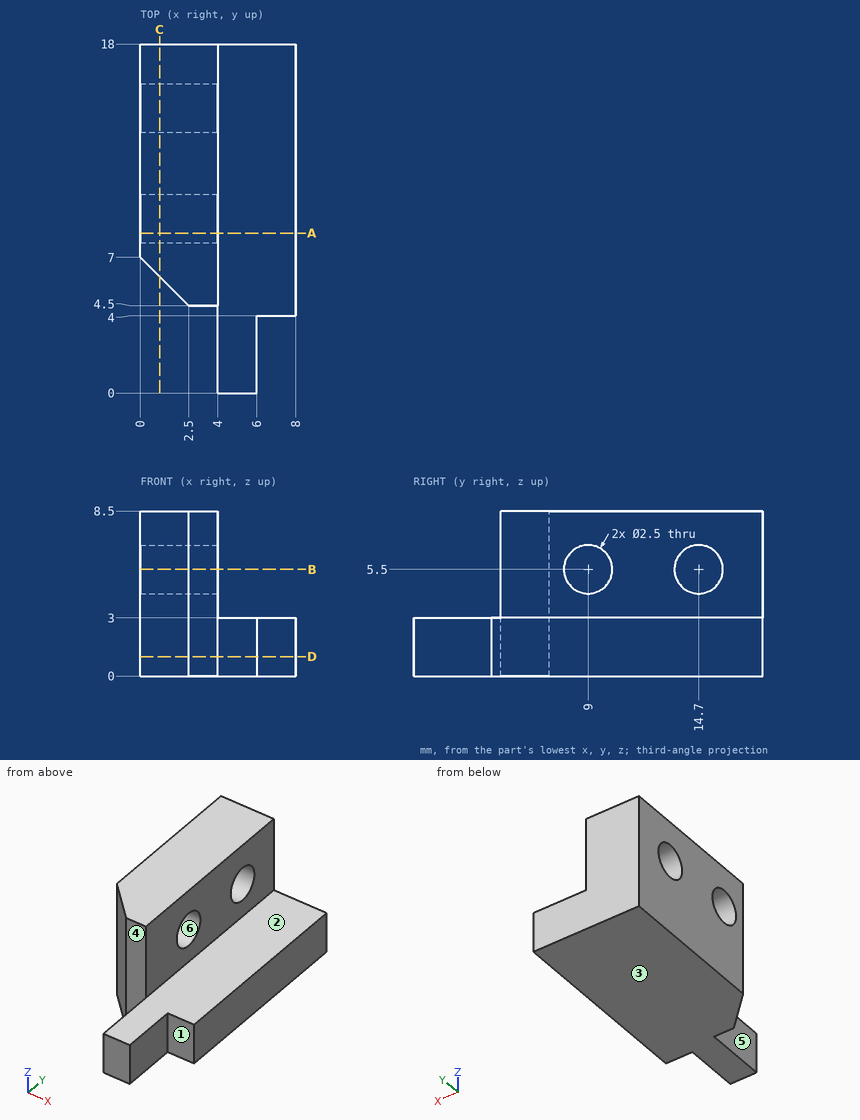
Part print with two shaded views. Sizes in mm from the minimum x, y, z corner. A direction names the side the tool comes from. Round coordinates to 2 decimals unless told otherwise and drop trailing zeros. Loops run counter-clockwise (first coordinate to the right, second up) from the corner with the lowest first, then second, coordinate; pieces in that order, holes last.
Item 1: Drill centre lines: line 1 along Y through (x, z) = (2.7, 5.5); line 2 along Y through (x, z) = (1, 5.5); line 3 along Y through (x, z) = (1, 2). Where is each one in solid material? Low to high.
Item 2: Which spindle directions (+Z, -Z, +X, -X, +Y, -Y) get a long thin tool onto all of the face, cutting with end or side? Do the marked faces 1, 2 and 3. Say none if no direction does.
Item 3: Saw through at A-A (y = 8.25). List the corners of the cut face in (x, z).
Item 4: Pin check, flat tips, straight feed: P1, Ø2.5, axis at y = 2.5, z = 1.5, coming from the +X side; P2, Ø0.8, axis at x = 3, z = 4.5, coming from the -Y side; P3, Ø2, axis at y = 9, z = 5.5, coming from the -X side; P4, Ø4.5, axis at y = 13.5, z = 7, coming from the +X side. Stop position of each tip, or through.
Item 5: Saw through at C-C (x = 1). List the corners of the cut face in (y, z).
Item 6: Two-plate mould, pull along Y, no slides. Class the marked faces 4, 5 and 6: released by +Y, released by -Y, zero draft, split by the parting line, or undercut.
Item 7: Saw through at B-B (z = 5.5). List the corners of the cut face in (x, y).
Item 8: Saw through at D-D (z = 1). List the corners of the cut face in (x, y), then the cut area to 3 significant figures.
Worked answers:
1. line 1: y = 4.5 to 7.75, 10.25 to 13.45, 15.95 to 18
1. line 2: y = 6 to 7.75, 10.25 to 13.45, 15.95 to 18
1. line 3: y = 6 to 18
2. face 1: +Z, -Z, +X, -Y
2. face 2: +Z, +X, +Y, -Y
2. face 3: -Z, +X, -X, +Y, -Y
3. outline: (0, 0) - (8, 0) - (8, 3) - (4, 3) - (4, 4.5) - (0, 4.5) - close; (0, 6.5) - (4, 6.5) - (4, 8.5) - (0, 8.5) - close
4. P1: stops at x = 6
4. P2: stops at y = 4.5
4. P3: passes through
4. P4: stops at x = 4
5. outline: (6, 0) - (18, 0) - (18, 8.5) - (6, 8.5) - close; hole circle Ø2.5 at (9, 5.5); hole circle Ø2.5 at (14.7, 5.5)
6. face 4: released by -Y
6. face 5: zero draft
6. face 6: undercut
7. outline: (0, 7) - (2.5, 4.5) - (4, 4.5) - (4, 7.75) - (0, 7.75) - close; (0, 10.25) - (4, 10.25) - (4, 13.45) - (0, 13.45) - close; (0, 15.95) - (4, 15.95) - (4, 18) - (0, 18) - close
8. outline: (0, 7) - (2.5, 4.5) - (4, 4.5) - (4, 0) - (6, 0) - (6, 4) - (8, 4) - (8, 18) - (0, 18) - close
8. area: 115 mm2
